from build123d import *

# Parameters (mm, degrees)
F0_W     = 286
F0_H     = 220
F1_DEPTH = 6.2
F2_W     = 5
F2_H     = 6.2
F2_W_2   = 12
F3_DEPTH = 6.2
F4_W     = 6.2
F4_H     = 12
F5_DEPTH = 6.2
F6_W     = 329.66836555
F6_H     = 26
F7_DEPTH = 6.201


with BuildPart() as f1:
    # F0 (on Top) → F1 (new body)
    with BuildSketch(Plane.XY):
        Rectangle(F0_W, F0_H)
    extrude(amount=F1_DEPTH)

    # F2 (on face) → F3 (join, through all)
    with BuildSketch(Plane.XY.offset(6.2)):
        with Locations((140.5, 113.1)):
            Rectangle(F2_W, F2_H)
        with Locations((120, 113.1)):
            Rectangle(F2_W_2, F2_H)
        with Locations((96, 113.1)):
            Rectangle(F2_W_2, F2_H)
        with Locations((72, 113.1)):
            Rectangle(F2_W_2, F2_H)
        with Locations((48, 113.1)):
            Rectangle(F2_W_2, F2_H)
        with Locations((24, 113.1)):
            Rectangle(F2_W_2, F2_H)
        with Locations((0, 113.1)):
            Rectangle(F2_W_2, F2_H)
        with Locations((-24, 113.1)):
            Rectangle(F2_W_2, F2_H)
        with Locations((-48, 113.1)):
            Rectangle(F2_W_2, F2_H)
        with Locations((-72, 113.1)):
            Rectangle(F2_W_2, F2_H)
        with Locations((-96, 113.1)):
            Rectangle(F2_W_2, F2_H)
        with Locations((-120, 113.1)):
            Rectangle(F2_W_2, F2_H)
        with Locations((-140.5, 113.1)):
            Rectangle(F2_W, F2_H)
    extrude(amount=-F3_DEPTH)

    # F4 (on face) → F5 (join, through all)
    with BuildSketch(Plane.XY.offset(6.2)):
        with Locations((146.1, -96)):
            Rectangle(F4_W, F4_H)
        with Locations((146.1, -72)):
            Rectangle(F4_W, F4_H)
        with Locations((146.1, -48)):
            Rectangle(F4_W, F4_H)
        with Locations((146.1, -24)):
            Rectangle(F4_W, F4_H)
        with Locations((146.1, 0)):
            Rectangle(F4_W, F4_H)
        with Locations((146.1, 24)):
            Rectangle(F4_W, F4_H)
        with Locations((146.1, 48)):
            Rectangle(F4_W, F4_H)
        with Locations((146.1, 72)):
            Rectangle(F4_W, F4_H)
        with Locations((146.1, 96)):
            Rectangle(F4_W, F4_H)
        with Locations((-146.1, 96)):
            Rectangle(F4_W, F4_H)
        with Locations((-146.1, 72)):
            Rectangle(F4_W, F4_H)
        with Locations((-146.1, 48)):
            Rectangle(F4_W, F4_H)
        with Locations((-146.1, 24)):
            Rectangle(F4_W, F4_H)
        with Locations((-146.1, 0)):
            Rectangle(F4_W, F4_H)
        with Locations((-146.1, -24)):
            Rectangle(F4_W, F4_H)
        with Locations((-146.1, -48)):
            Rectangle(F4_W, F4_H)
        with Locations((-146.1, -72)):
            Rectangle(F4_W, F4_H)
        with Locations((-146.1, -96)):
            Rectangle(F4_W, F4_H)
    extrude(amount=-F5_DEPTH)

    # F6 (on face) → F7 (cut, through all)
    with BuildSketch(Plane.XY.offset(6.2)):
        with Locations((15.634182775, -97)):
            Rectangle(F6_W, F6_H)
    extrude(amount=-F7_DEPTH, mode=Mode.SUBTRACT)


solid = f1.part
Model file for the job. Use its own axes, mm. A direction names the side the tool comes from. Round coordinates to 2 decimals unless told otherwise and drop trailing zeros. Loops run counter-clockwise (first coordinate to the right, second up) from the corner with the lowest first, then second, coordinate; pieces in that order, holes last. Notation, with made-up numbers: (34.25, 38) - (92.25, 38) arc R19 cw to (92.25, 43) - close; hole circle Ø1 at (88, 0). An arc over 180 degrees is marked (long way). Write each question's results on one line, items separated by ' | '.
(1) Wall check: L1, parallel to Y at x = 10, z = 0.75; L2, parallel to X at y = 103, z = 1. Give the ranges that are in metal, low to high.
Answer below:
L1: y = -84 to 110 | L2: x = -143 to 143
(2) Saw through at A-A, the plane y = 62.5. List the corners of the cut face in (x, z), then the cut area to 3 significant figures.
Answer below:
outline: (-143, 0) - (143, 0) - (143, 6.2) - (-143, 6.2) - close | area: 1,770 mm^2
(3) Saw through at B-B, the plane x = 106. List the corners of the cut face in (y, z), then the cut area to 3 significant figures.
Answer below:
outline: (-84, 0) - (110, 0) - (110, 6.2) - (-84, 6.2) - close | area: 1,200 mm^2
(4) Pin check, flat tips, straight feed: pin 1 (3 mm diameter, centred on x = -10, z = 2, fed in from +Y); pin 2 (1.9 mm diameter, centred on y = 113, z = 4, fed in from -X); pin 3 (1.9 mm diameter, centred on x = 145, z = 2.5, fed in from +Y). Stop position of each tip, or through.
Answer below:
pin 1: stops at y = 110 | pin 2: stops at x = -143 | pin 3: stops at y = 102
(5) Mould opens along X. For faces 1 (the flat face through (-48, 116.2, 3)), 2 (the flat face through (-143, 36, 3)), 3 (the flat face through (102, 113, 3)), 4 (the flat face through (-138, 113, 3)) say: released by +X, released by -X, zero draft, split by the parting line, or undercut.
Answer below:
face 1: zero draft | face 2: released by -X | face 3: undercut | face 4: undercut
(6) 3-axis set-ups, long thin cutter, end or side, ignore diameter. For faces 5 (the flat face through (-102, 113, 3)), 6 (the flat face through (146, -30, 3)), 7 (the flat face through (-2, 18, 0)), 8 (the flat face through (-146, 6, 3)): which of +Z, -Z, +X, -X, +Y, -Y reach the whole face in a straight line?
Answer below:
face 5: +Z, -Z, +Y | face 6: +Z, -Z, +X | face 7: -Z, +X, -X, +Y, -Y | face 8: +Z, -Z, -X
